Part model, mm, in its own coordinate system. Give positions to 0.01 mm unless a question says otherwise; leave off trailing zeros. Order: outer loops, then holes, each group sorted by start corner. A loop starts at its lowest first (then second) coordinate and runs counter-clockwise, first axis right, second up.
from build123d import *

# Parameters (mm, degrees)
SKETCH1_W               = 323
SKETCH1_H               = 50
BOSS_EXTRUDE1_DEPTH     = 3
SKETCH2_W               = 70
SKETCH2_H               = 40
CUT_EXTRUDE1_DEPTH      = 1
CUT_EXTRUDE1_DEPTH_BACK = 4
FILLET1_R               = 2
SKETCH3_W               = 323
SKETCH3_H               = 3
BOSS_EXTRUDE2_DEPTH     = 2.5
SKETCH4_R               = 1.75
CUT_EXTRUDE2_DEPTH      = 4


with BuildPart() as part:
    # Sketch1 → Boss-Extrude1 (new body)
    with BuildSketch(Plane.XY):
        Rectangle(SKETCH1_W, SKETCH1_H)
    extrude(amount=BOSS_EXTRUDE1_DEPTH)

    # Sketch2 → Cut-Extrude1 (cut, two sides)
    with BuildSketch(Plane.XY.offset(3)) as cut_extrude1_sk:
        with Locations((0, -5)):
            Rectangle(SKETCH2_W, SKETCH2_H)
    extrude(amount=CUT_EXTRUDE1_DEPTH, mode=Mode.SUBTRACT)
    extrude(cut_extrude1_sk.sketch, amount=-CUT_EXTRUDE1_DEPTH_BACK, mode=Mode.SUBTRACT)

    # Fillet1
    fillet1_edges = [part.edges().sort_by_distance(p)[0] for p in [
        (-35, 15, 1.5),
        (35, 15, 1.5),
    ]]
    fillet(fillet1_edges, radius=FILLET1_R)

    # Sketch3 → Boss-Extrude2 (add)
    with BuildSketch(Plane(origin=(0, 25, 0), x_dir=(1, 0, 0), z_dir=(0, 1, 0))):
        with Locations((0, -1.5)):
            Rectangle(SKETCH3_W, SKETCH3_H)
    extrude(amount=BOSS_EXTRUDE2_DEPTH)

    # Sketch4 → Cut-Extrude2 (cut, through all)
    with BuildSketch(Plane.XY.offset(3)):
        with Locations((-152.5, -5)):
            Circle(SKETCH4_R)
        with Locations(Location((152.5, -5, 0), (0, 0, 180))):  # turned: the seam where the file's is
            Circle(SKETCH4_R)
    extrude(amount=-CUT_EXTRUDE2_DEPTH, mode=Mode.SUBTRACT)


solid = part.part
Item 1: Band-saw the part on A-A on y = 8.5. List the corners of the cut face in (x, z).
Item 2: Drill centre lines: probe 1 along X at (y, z) = (3.5, 0.45); probe 2 along Y at (x, z) = (152.5, 1.4); probe 3 along Y at (x, z) = (27, 2.5). Where is each one in solid material? Low to high.
Item 3: Band-saw the part on B-B on z = 1.3. List the corners of the cut face in (x, y).
Working result:
1. outline: (-161.5, 0) - (-35, 0) - (-35, 3) - (-161.5, 3) - close; (35, 0) - (161.5, 0) - (161.5, 3) - (35, 3) - close
2. probe 1: x = -161.5 to -35, 35 to 161.5
2. probe 2: y = -25 to -6.75, -3.25 to 27.5
2. probe 3: y = 15 to 27.5
3. outline: (-161.5, -25) - (-35, -25) - (-35, 13) arc R2 cw to (-33, 15) - (33, 15) arc R2 cw to (35, 13) - (35, -25) - (161.5, -25) - (161.5, 27.5) - (-161.5, 27.5) - close; hole circle Ø3.5 at (-152.5, -5); hole circle Ø3.5 at (152.5, -5)
